from build123d import *

# Parameters (mm, degrees)
BOSS_EXTRUDE1_DEPTH          = 1.5
M3_CLEARANCE_HOLE1_D         = 3.2
F_1_8_0_125_DIAMETER_HOLE1_D = 3.175
M3_CLEARANCE_HOLE2_D         = 3.2
CUT_EXTRUDE1_DEPTH           = 151.461996863
SKETCH11_R                   = 0.5
CUT_EXTRUDE2_DEPTH           = 151.108502424


with BuildPart() as part:
    # Sketch1 → Boss-Extrude1 (new body)
    with BuildSketch(Plane.XY):
        with BuildLine():
            Line((0, 0), (0, 60))
            Line((0, 60), (-70.75, 60))
            ThreePointArc((-70.75, 60), (-94.79163056, 50.04163056), (-104.75, 26))
            Line((-104.75, 26), (-104.75, -106))
            ThreePointArc((-104.75, -106), (-104.164213562, -107.414213562), (-102.75, -108))
            Line((-102.75, -108), (-48.25, -108))
            ThreePointArc((-48.25, -108), (-46.835786438, -107.414213562), (-46.25, -106))
            Line((-46.25, -106), (-46.25, -13))
            ThreePointArc((-46.25, -13), (-42.442388155, -3.807611845), (-33.25, 0))
            Line((-33.25, 0), (0, 0))
        make_face()
    extrude(amount=BOSS_EXTRUDE1_DEPTH)

    # Mirror1: part across plane


with BuildPart() as part_1:
    add(part.part)
    add(part.part.mirror(Plane(origin=(0, 0, 0), x_dir=(0, 0, 1), z_dir=(1, 0, 0))))

    # M3 Clearance Hole1 (through all)
    with Locations(Plane(origin=(0, 0, 0), x_dir=(-1, 0, 0), z_dir=(0, 0, -1))):
        with Locations((0, 57.25), (78, 56.25), (81.25, 47.5), (81.75, 5.5), (101, -27.75), (43, -0.75), (50.9757, -73.488), (57.8845, -103.079), (98.5499, -81.5652), (98.5499, -103.079), (-100.0866, -73.488), (-93.1778, -103.079), (-52.5124, -81.5652), (-52.5124, -103.079), (-43, -0.75), (-101, -27.75), (-81.75, 5.5), (-81.25, 47.5), (-78, 56.25)):
            Hole(M3_CLEARANCE_HOLE1_D / 2)

    # 1/8 (0.125) Diameter Hole1 (through all)
    with Locations(Plane(origin=(0, 0, 0), x_dir=(-1, 0, 0), z_dir=(0, 0, -1))):
        with Locations((-100.0104, -88.1946), (-52.5124, -88.1946), (51.0519, -88.1946), (98.5499, -88.1946)):
            Hole(F_1_8_0_125_DIAMETER_HOLE1_D / 2)

    # M3 Clearance Hole2 (through all)
    with Locations(Plane(origin=(0, 0, 0), x_dir=(-1, 0, 0), z_dir=(0, 0, -1))):
        with Locations((-57.5, 48.5), (-57.5, 11.5), (57.5, 48.5), (57.5, 11.5)):
            Hole(M3_CLEARANCE_HOLE2_D / 2)

    # Sketch10 → Cut-Extrude1 (cut, through all)
    with BuildSketch(Plane(origin=(0, 0, 0), x_dir=(-1, 0, 0), z_dir=(0, 0, -1))):
        with BuildLine():
            Line((-70.75, 60), (70.75, 60))
            ThreePointArc((70.75, 60), (94.79163056, 50.04163056), (104.75, 26))
            Line((104.75, 26), (104.75, -106))
            ThreePointArc((104.75, -106), (104.164213562, -107.414213562), (102.75, -108))
            Line((102.75, -108), (48.25, -108))
            ThreePointArc((48.25, -108), (46.835786438, -107.414213562), (46.25, -106))
            Line((46.25, -106), (46.25, -13))
            ThreePointArc((46.25, -13), (42.442388155, -3.807611845), (33.25, 0))
            Line((33.25, 0), (-33.25, 0))
            ThreePointArc((-33.25, 0), (-42.442388155, -3.807611845), (-46.25, -13))
            Line((-46.25, -13), (-46.25, -106))
            ThreePointArc((-46.25, -106), (-46.835786438, -107.414213562), (-48.25, -108))
            Line((-48.25, -108), (-102.75, -108))
            ThreePointArc((-102.75, -108), (-104.164213562, -107.414213562), (-104.75, -106))
            Line((-104.75, -106), (-104.75, 26))
            ThreePointArc((-104.75, 26), (-94.79163056, 50.04163056), (-70.75, 60))
        make_face()
        with BuildLine():
            Line((-70.75, 59.75), (70.75, 59.75))
            ThreePointArc((70.75, 59.75), (94.614853865, 49.864853865), (104.5, 26))
            Line((104.5, 26), (104.5, -106))
            ThreePointArc((104.5, -106), (103.987436867, -107.237436867), (102.75, -107.75))
            Line((102.75, -107.75), (48.25, -107.75))
            ThreePointArc((48.25, -107.75), (47.012563133, -107.237436867), (46.5, -106))
            Line((46.5, -106), (46.5, -13))
            ThreePointArc((46.5, -13), (42.619164851, -3.630835149), (33.25, 0.25))
            Line((33.25, 0.25), (-33.25, 0.25))
            ThreePointArc((-33.25, 0.25), (-42.619164851, -3.630835149), (-46.5, -13))
            Line((-46.5, -13), (-46.5, -106))
            ThreePointArc((-46.5, -106), (-47.012563133, -107.237436867), (-48.25, -107.75))
            Line((-48.25, -107.75), (-102.75, -107.75))
            ThreePointArc((-102.75, -107.75), (-103.987436867, -107.237436867), (-104.5, -106))
            Line((-104.5, -106), (-104.5, 26))
            ThreePointArc((-104.5, 26), (-94.614853865, 49.864853865), (-70.75, 59.75))
        make_face(mode=Mode.SUBTRACT)
    extrude(amount=-CUT_EXTRUDE1_DEPTH, mode=Mode.SUBTRACT)

    # Sketch11 → Cut-Extrude2 (cut, through all)
    with BuildSketch(Plane(origin=(0, 0, 0), x_dir=(-1, 0, 0), z_dir=(0, 0, -1))):
        with Locations((-60, -12.5)):
            Circle(SKETCH11_R)
        with Locations((-62.5, -54.44375)):
            Circle(SKETCH11_R)
        with Locations((59, -56.0874)):
            Circle(SKETCH11_R)
        with Locations((62.25, -12.5)):
            Circle(SKETCH11_R)
        with Locations((-63.8789, -94.9764)):
            Circle(SKETCH11_R)
        with Locations((87.1961, -94.9764)):
            Circle(SKETCH11_R)
        with Locations((50.02, 10.5)):
            Circle(SKETCH11_R)
    extrude(amount=-CUT_EXTRUDE2_DEPTH, mode=Mode.SUBTRACT)


solid = part_1.part
Can you work these out from the model? Positions are in its coordinate system, mm. A direction names the side the tool comes from. Round coordinates to 2 decimals unless told otherwise and drop trailing zeros. Write each loop counter-clockwise with the first axis right and the second up, starting at its lowest first coordinate (ties: lowest second). Pieces come first, ordered by that corner, then holes. Notation, with made-up numbers: M -36.75,60 L -1.75,60 A31 ccw -1.75,97 Z; hole C 63,8 d9. An arc over 180 degrees is marked long. Use a Markdown table: item, result.
Item 1: I want a section at B-B (z = 0.6). State how many separate pieces and enclosed holes the cut face has, and give its area (3 significant figures).
Found:
| item | result |
|---|---|
| separate pieces | 1 |
| enclosed holes | 34 |
| area | 24,300 mm2 |
Item 2: Which directions (+Z, -Z, +X, -X, +Y, -Y) give clear straight access to the entire face, cutting with the end or side of a thin tool? Please do faces 4 (the face through (-94.351, 50.126, 0.74)), 5 (the face through (42.52, -3.53, 0.74)).
Found:
| item | result |
|---|---|
| face 4 | +Z, -Z, -X, +Y |
| face 5 | +Z, -Z, -Y |
Item 3: I want a section at A-A (y = -9.5). List the corners of the cut face in (x, z) for me.
Found:
| item | result |
|---|---|
| outline | M -104.5,0 L -46.03,0 L -46.03,1.5 L -104.5,1.5 Z; M 46.03,0 L 104.5,0 L 104.5,1.5 L 46.03,1.5 Z |
Item 4: For pin 1 Ø5 at (x, y) = (57.5, 11.5) entering from -Z, with a flat end and sliding along its axis, tell me the tip position at first contact or that it passes through.
Found:
| item | result |
|---|---|
| pin 1 | stops at z = 0 |
Item 5: We'd pull the mould along X, two halves only. Please class faces 1 (the face through (-42.72, -3.73, 0.74)), 2 (the face through (1, 14, 1.5)), 3 (the face through (94.876, 49.601, 0.74)): released by +X, released by -X, zero draft, split by the parting line, or undercut.
Found:
| item | result |
|---|---|
| face 1 | undercut |
| face 2 | zero draft |
| face 3 | released by +X |
Item 6: If I drill on line 1 along Y through (x, z) = (57.5, 1.25); line 2 along X through (y, z) = (-92, 1.25); line 3 along X through (y, z) = (5, 0.1), over which ranges is the centre line in solid material (lowest first)? Write a range as [from, to].
Found:
| item | result |
|---|---|
| line 1 | y = [-107.75, 9.9], [13.1, 46.9], [50.1, 59.75] |
| line 2 | x = [-104.5, -46.5], [46.5, 104.5] |
| line 3 | x = [-104.5, -83.27], [-80.23, 80.23], [83.27, 104.5] |
